Design review of the part built by this model. Coordinates are the model's own, in mm. Face numbers are marked on the shaded views. A direction names the side the tool comes from. Round coordinates to 2 decimals unless told otherwise and drop trailing zeros. Loops run counter-clockwise (first coordinate to the right, second up) from the corner with the lowest first, then second, coordinate; pieces in that order, holes last. Notation, with made-up numbers: (21, 18.25) -> (78, 18.25) arc R22 ccw to (78, 33.25) -> close; hole circle Ø5 at (-38.75, 30). An arc over 180 degrees is marked (long way). Answer as CSV lines item,"result". Start each with the question number.
```python
from build123d import *

# Parameters (mm, degrees)
CORTAR_EXTRUIR1_DEPTH = 2.5


with BuildPart() as part:
    # Croquis1 → Revolución1 (revolve)
    with BuildSketch(Plane(origin=(0, 0, 0), x_dir=(0, 0, -1), z_dir=(1, 0, 0)), mode=Mode.PRIVATE) as revoluci_n1_sk:
        Polygon((0, 0), (15, 0), (15, 2), (14.5, 2.5), (1.945299462, 2.5), (1.345299462, 2.541956087), (1.345299462, 4.125), (1.220299462, 4.25), (-3.154700538, 4.25), (-3.654700538, 3.75), (-3.654700538, 2.3), (-3.354700538, 2), (-1.154700538, 2), align=None)
    revolve(revoluci_n1_sk.sketch.rotate(Axis((0, 0, 0), (0, 0, -1)), 90), axis=Axis((0, 0, 0), (0, 0, -1)))

    # Croquis2 → Cortar-Extruir1 (cut)
    with BuildSketch(Plane.XY.offset(3.654700538)):
        Polygon((0, 2.309401077), (-2, 1.154700538), (-2, -1.154700538), (0, -2.309401077), (2, -1.154700538), (2, 1.154700538), align=None)
    extrude(amount=-CORTAR_EXTRUIR1_DEPTH, mode=Mode.SUBTRACT)


solid = part.part
```
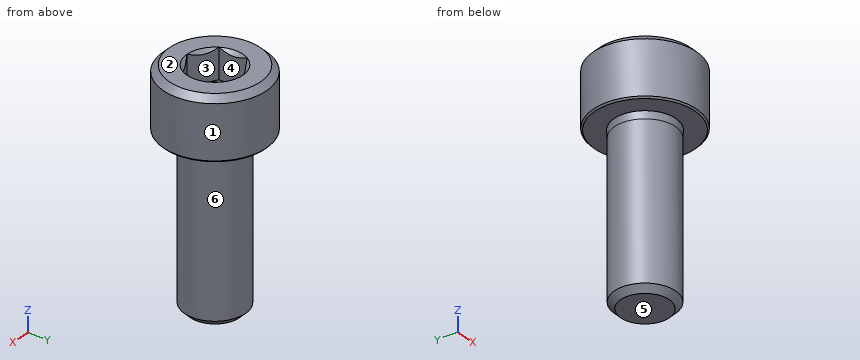
Q1. Machinability: for the marked faces 5 and 6, which of the approach directions +Z, -Z, +X, -X, +Y, -Y give a long, thin tool a straight path to every point of the face, cutting with its end or side? Answer none if there is none.
Q2. To check wall thickness, follow probe 1 along Z at (x, y) = (1.25, -2.5); probe 2 along X at (y, z) = (-1.5, -11.5); probe 3 along X at (y, z) = (0.5, 2.25). State the ranges of each line that lie inside material, in increasing order. Write a range as from..to.
Q3. For pin 1 Ø1 at (y, z) = (0.5, -9.5) entering from -X; pin 2 Ø4 at (y, z) = (2.5, -7) entering from -X; pin 3 Ø0.5 at (x, y) = (1.5, 0.5) entering from +Z, all flat-tipped, find the tip position at first contact; note any pin that passes through.
Q4. Mouldability with a two-part tool opening along X and no side actions: class the marked faces 1, 2, 3 and 4 as pulls with the +X half, pulls with the -X half, needs draft (parallel to the pull), parting line crosses it, or undercut.
Q5. Add section A-A, the plane z = -7.75. Give the boundary of the cut face in (x, y).
Worked answers:
1,face 5,"-Z, +X, -X, +Y, -Y"
1,face 6,"-Z"
2,probe 1,"z = -1.35..3.65"
2,probe 2,"x = -2..2"
2,probe 3,"x = -4.22..-2, 2..4.22"
3,pin 1,"stops at x = -2.5"
3,pin 2,"stops at x = -2.45"
3,pin 3,"stops at z = 1.06"
4,face 1,"parting line crosses it"
4,face 2,"needs draft"
4,face 3,"undercut"
4,face 4,"undercut"
5,outline,"circle Ø5 at (0, 0)"
